Check sheet for the modelled part. Datum: model origin and axes. Units: mm. Face numbers are marked on the shaded views. A direction names the side the tool comes from. Round coordinates to 2 decimals unless told otherwise and drop trailing zeros. Order: outer loops, then holes, each group sorted by start corner. A loop starts at its lowest first (then second) coordinate and runs counter-clockwise, first axis right, second up.
```python
from build123d import *

# Parameters (mm, degrees)
SKETCH1_R           = 1.75
BOSS_EXTRUDE1_DEPTH = 48
CUT_EXTRUDE1_DEPTH  = 44
BOSS_EXTRUDE2_START = -10
BOSS_EXTRUDE2_DEPTH = 10
CUT_EXTRUDE2_START  = -10
CUT_EXTRUDE2_DEPTH  = 10
FILLET3_R           = 1
SKETCH6_R           = 1.75
CUT_EXTRUDE3_DEPTH  = 10


with BuildPart() as part:
    # Sketch1 → Boss-Extrude1 (new body)
    with BuildSketch(Plane(origin=(0, 0, 0), x_dir=(1, 0, 0), z_dir=(0, 1, 0))):
        with BuildLine():
            Line((-5, 4.5), (5, 4.5))
            ThreePointArc((5, 4.5), (9.5, 0), (5, -4.5))
            Line((5, -4.5), (-5, -4.5))
            ThreePointArc((-5, -4.5), (-9.5, 0), (-5, 4.5))
        make_face()
        with Locations(Location((-5, 0, 0), (0, 0, 270))):
            Circle(SKETCH1_R, mode=Mode.SUBTRACT)
        with Locations(Location((5, 0, 0), (0, 0, 270))):
            Circle(SKETCH1_R, mode=Mode.SUBTRACT)
    extrude(amount=BOSS_EXTRUDE1_DEPTH)

    # Sketch2 → Cut-Extrude1 (cut)
    with BuildSketch(Plane(origin=(0, 48, 0), x_dir=(1, 0, 0), z_dir=(0, 1, 0))):
        Polygon((-1.651368439, 0), (-3.325684219, 2.9), (-6.674315781, 2.9), (-8.348631561, 0), (-6.674315781, -2.9), (-3.325684219, -2.9), align=None)
        Polygon((3.325684219, -2.9), (1.651368439, 0), (3.325684219, 2.9), (6.674315781, 2.9), (8.348631561, 0), (6.674315781, -2.9), align=None)
    extrude(amount=-CUT_EXTRUDE1_DEPTH, mode=Mode.SUBTRACT)

    # Sketch4 → Boss-Extrude2 (add)
    with BuildSketch(Plane(origin=(0, 48, 0), x_dir=(1, 0, 0), z_dir=(0, 1, 0)).offset(BOSS_EXTRUDE2_START)):
        with BuildLine():
            Line((-5, -4.5), (5, -4.5))
            ThreePointArc((5, -4.5), (7.342329219, -3.842329219), (9, -2.061552813))
            Line((9, -2.061552813), (9, -6))
            Line((9, -6), (29.5, -6))
            Line((29.5, -6), (29.5, -8.5))
            Line((29.5, -8.5), (10.5, -8.5))
            Line((10.5, -8.5), (-10.5, -8.5))
            Line((-10.5, -8.5), (-29.5, -8.5))
            Line((-29.5, -8.5), (-29.5, -6))
            Line((-29.5, -6), (-9, -6))
            Line((-9, -6), (-9, -2.061552813))
            ThreePointArc((-9, -2.061552813), (-7.342329219, -3.842329219), (-5, -4.5))
        make_face()
    extrude(amount=BOSS_EXTRUDE2_DEPTH)

    # Sketch5 → Cut-Extrude2 (cut)
    with BuildSketch(Plane(origin=(0, 48, 0), x_dir=(1, 0, 0), z_dir=(0, 1, 0)).offset(CUT_EXTRUDE2_START)):
        with BuildLine():
            Line((-9.5, 0), (9.5, 0))
            ThreePointArc((9.5, 0), (8.181980515, 3.181980515), (5, 4.5))
            Line((5, 4.5), (-5, 4.5))
            ThreePointArc((-5, 4.5), (-8.181980515, 3.181980515), (-9.5, 0))
        make_face()
    extrude(amount=CUT_EXTRUDE2_DEPTH, mode=Mode.SUBTRACT)

    # Fillet3
    fillet3_edges = [part.edges().sort_by_distance(p)[0] for p in [
        (-9, 43, 6),
        (-9, 43, 2.061552813),
        (9, 43, 2.061552813),
        (9, 43, 6),
    ]]
    fillet(fillet3_edges, radius=FILLET3_R)

    # Sketch6 → Cut-Extrude3 (cut)
    with BuildSketch(Plane.XY.offset(8.5)):
        with Locations((-25, 43)):
            Circle(SKETCH6_R)
        with Locations((25, 43)):
            Circle(SKETCH6_R)
    extrude(amount=-CUT_EXTRUDE3_DEPTH, mode=Mode.SUBTRACT)


solid = part.part
```
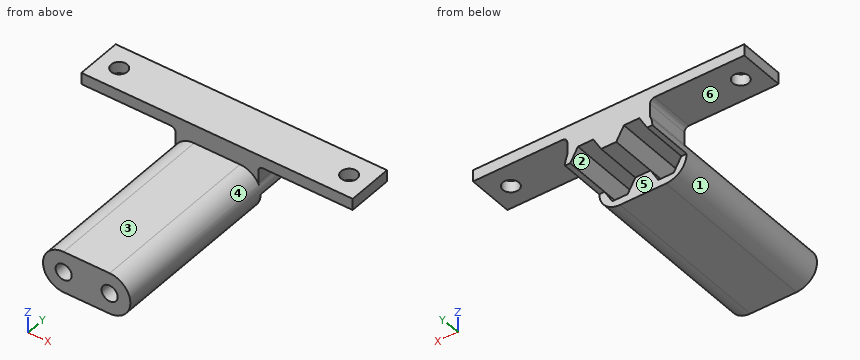
Item 1: Sectioned sample at C-C (z = 7.75). Record the cut outline in (x, y), and give its area (3 significant figures).
Answer:
outline: (-29.5, 38) - (29.5, 38) - (29.5, 48) - (-29.5, 48) - close; hole circle Ø3.5 at (-25, 43); hole circle Ø3.5 at (25, 43)
area: 571 mm2
Item 2: Access from +Z, -Z, +X, -X, +Y, -Y to the whole of each face (thin tool, end or side, straight path). Record for the marked faces 4, 5 and 6.
Answer:
face 4: +X, -Y
face 5: -Z, +X, -X, +Y
face 6: -Z, -X, +Y, -Y
Item 3: Go/stop test with flat-tipped pins: P1, Ø3, axis at x = 5.5, z = 0.5, coming from the +Y side; P2, Ø3.5, axis at x = -7.5, z = 6.5, coming from the -Y side; P3, Ø1, axis at x = 6, y = 35, coming from the -Z side; P4, Ø2, axis at x = 25, y = 43, coming from the -Z side. Record where each tip stops, or that it passes through.
Answer:
P1: stops at y = 4
P2: stops at y = 38
P3: stops at z = -4.47
P4: passes through
Item 4: Sectioned sample at D-D (y = 44). State how many separate pieces and enclosed holes the cut face has, and give its area (3 significant figures).
Answer:
separate pieces: 3
enclosed holes: 0
area: 214 mm2
Item 5: Sectioned sample at B-B (y = 9.5). Record the cut outline in (x, z), and give its area (3 significant figures).
Answer:
outline: (-5, -4.5) - (5, -4.5) arc R4.5 ccw to (5, 4.5) - (-5, 4.5) arc R4.5 ccw to start; hole (-8.35, 0) - (-6.67, -2.9) - (-3.33, -2.9) - (-1.65, 0) - (-3.33, 2.9) - (-6.67, 2.9) - close; hole (1.65, 0) - (3.33, -2.9) - (6.67, -2.9) - (8.35, 0) - (6.67, 2.9) - (3.33, 2.9) - close
area: 95.4 mm2
Item 6: Release check for a two-part mould opening along X. For the marked faces 1, 2 and 3 record: released by +X, released by -X, zero draft, split by the parting line, or undercut.
Answer:
face 1: released by -X
face 2: undercut
face 3: zero draft
Item 7: Sectioned sample at A-A (x = -25). Record the cut outline in (y, z), and give its area (4 significant figures).
Answer:
outline: (38, 6) - (41.25, 6) - (41.25, 8.5) - (38, 8.5) - close; (44.75, 6) - (48, 6) - (48, 8.5) - (44.75, 8.5) - close
area: 16.25 mm2
Item 8: Scan lines: line 1 along X through (y, z) = (1.2, 0); line 2 along Z through (x, y) = (-5, 1.7); line 3 along X through (y, z) = (37, -1.75). Record each from-to range of solid material in increasing order.
Answer:
line 1: x = -9.5 to -6.75, -3.25 to 3.25, 6.75 to 9.5
line 2: z = -4.5 to -1.75, 1.75 to 4.5
line 3: x = -9.15 to -7.34, -2.66 to 2.66, 7.34 to 9.15
